from build123d import *

# Parameters (mm, degrees)
F1_DEPTH = 12.5
F2_W     = 8.6661115155
F2_H     = 37.1920648861
F2_W_2   = 11.7714676749
F2_H_2   = 37.3365031319
F3_DEPTH = 25
F4_W     = 10.3762667931
F4_H     = 26.0754239581
F4_W_2   = 12.8692660095
F4_H_2   = 27.2882347388
F5_DEPTH = 25


with BuildPart() as f1:
    # F0 (on Front) → F1 (new body, symmetric)
    with BuildSketch(Plane.XZ):
        with BuildLine():
            ThreePointArc((113.5, 0), (0, -113.5), (-113.5, 0))
            Line((-113.5, 0), (-138.5, 0))
            Line((-138.5, 0), (-163.5, 0))
            Line((-163.5, 0), (-163.5, -12))
            Line((-163.5, -12), (-137.9791650939, -12))
            ThreePointArc((-137.9791650939, -12), (0.3305438412, -138.4996055618), (138.0348714685, -11.3412635401))
            Line((138.0348714685, -11.3412635401), (163.5, -11))
            Line((163.5, -11), (163.5, 0))
            Line((163.5, 0), (158.027844932, 0))
            ThreePointArc((158.027844932, 0), (155.5, -0.9), (152.972155068, 0))
            Line((152.972155068, 0), (147.5, 0))
            Line((147.5, 0), (138.5, 0))
            Line((138.5, 0), (113.5, 0))
        make_face()
        with BuildLine():
            Line((147.5, 7), (147.5, 0))
            Line((147.5, 0), (152.972155068, 0))
            ThreePointArc((152.972155068, 0), (153.7841007792, 6.7132658169), (159.5, 3.1))
            ThreePointArc((159.5, 3.1), (159.1132658169, 1.3841007792), (158.027844932, 0))
            Line((158.027844932, 0), (163.5, 0))
            Line((163.5, 0), (163.5, 7))
            ThreePointArc((163.5, 7), (155.5, 12), (147.5, 7))
        make_face()
    extrude(amount=F1_DEPTH, both=True)

    # F2 (on face) → F3 (cut)
    with BuildSketch(Plane.YZ.offset(163.5)):
        with Locations((-10.3330557577, -0.399579161)):
            Rectangle(F2_W, F2_H)
        with Locations((11.8857338375, -1.6272780021)):
            Rectangle(F2_W_2, F2_H_2)
    extrude(amount=-F3_DEPTH, mode=Mode.SUBTRACT)

    # F4 (on face) → F5 (cut)
    with BuildSketch(Plane(origin=(-163.5, 0, 0), x_dir=(0, -1, 0), z_dir=(-1, 0, 0))):
        with Locations((-11.1881333965, -6.0408366425)):
            Rectangle(F4_W, F4_H)
        with Locations((12.4346330048, -6.9841346379)):
            Rectangle(F4_W_2, F4_H_2)
    extrude(amount=-F5_DEPTH, mode=Mode.SUBTRACT)


solid = f1.part
Check sheet for the modelled part. Datum: model origin and axes. Units: mm. A direction names the side the tool comes from. Give positions to 0.01 mm unless a question says otherwise; leave off trailing zeros. Write each loop counter-clockwise with the first axis right and the second up, starting at its lowest first coordinate (ties: lowest second). Pieces come first, ordered by that corner, then holes. Notation, with made-up numbers: (55.5, 32) -> (89.5, 32) arc R17 cw to (89.5, 51) -> close; hole circle Ø10 at (-19, -25). An arc over 180 degrees is marked (long way). Use one line per item in the form item = value. Start each with the question number.
1. Section check C-C (x = 155.5). Record the cut outline in (y, z).
2. Go/stop test with flat-tipped pins: P1, Ø12, axis at y = -1, z = -82.5, coming from the +X side; P2, Ø13, axis at x = -153.5, z = -3.5, coming from the -Y side; P3, Ø1.5, axis at y = -1.5, z = -74.5, coming from the +X side; P4, Ø7, axis at y = -8.5, z = -6, coming from the +X side. Record where each tip stops, or that it passes through.
3. Section check D-D (x = 0). Record the cut outline in (y, z), and give its area (3 significant figures).
4. Thickness scan on line 1 along Z through (x, y) = (142.5, 0.5); line 2 along X through (y, z) = (-9, -67); line 3 along X through (y, z) = (-1.75, -85.5). Record the ranges inside material, lowest first. Write a range as from..to.
5. Access from +Z, -Z, +X, -X, +Y, -Y to the whole of each face (thin tool, end or side, straight path). Record for faces 1 (the flat face through (-133, 0, 0)), 2 (the flat face through (-151, 6, -6)), 3 (the flat face through (138.5, 9, -6)), 4 (the flat face through (-151, -6, -6)), 5 (the flat face through (138.5, -9, -6)).
6. Section check A-A (z = 3.1). Record the cut outline in (x, y).
7. Section check B-B (y = -2.75). Record the cut outline in (x, z), and give its area (3 significant figures).
Conclusion:
q1.outline = (-6, -11.11) -> (6, -11.11) -> (6, -0.9) -> (-6, -0.9) -> close; (-6, 7.1) -> (6, 7.1) -> (6, 12) -> (-6, 12) -> close
q2.P1 = 115.46
q2.P2 = -6
q2.P3 = 117.23
q2.P4 = 163.5
q3.outline = (-12.5, -138.5) -> (12.5, -138.5) -> (12.5, -113.5) -> (-12.5, -113.5) -> close
q3.area = 625 mm²
q4.line_1 = -11.28..0
q4.line_2 = -121.22..-91.61, 91.61..121.22
q4.line_3 = -108.96..-74.65, 74.65..108.96
q5.face_1 = +Z, -X, +Y, -Y
q5.face_2 = +Z, -Z, -X, +Y
q5.face_3 = +Z, -Z, +X, +Y
q5.face_4 = +Z, -Z, -X, -Y
q5.face_5 = +Z, -Z, +X, -Y
q6.outline = (147.5, -6) -> (151.5, -6) -> (151.5, 6) -> (147.5, 6) -> close; (159.5, -6) -> (163.5, -6) -> (163.5, 6) -> (159.5, 6) -> close
q7.outline = (-163.5, -12) -> (-137.98, -12) arc R138.5 ccw to (138.03, -11.34) -> (163.5, -11) -> (163.5, 7) arc R8.9 ccw to (147.5, 7) -> (147.5, 0) -> (113.5, 0) arc R113.5 cw to (-113.5, 0) -> (-163.5, 0) -> close; hole circle Ø8 at (155.5, 3.1)
q7.area = 10,600 mm²
